The listing builds one solid part. Answer for the finished solid, in the listing's coordinates (mm). Coordinates: 2 decimals unless noted, no trailing zeros. Order: outer loops, then holes, each group sorted by start corner. A loop starts at its lowest first (then second) coordinate and runs counter-clockwise, first axis right, second up. Notation, with made-up numbers: (47.25, 84.25) - (96.25, 84.25) arc R14 cw to (96.25, 104.25) - close; hole circle Ø10 at (64, 74.5). An arc over 180 degrees is marked (long way). Use one line per item in the form item = value. Start each with the question number.
Item 1: Section B-B, the plane x = -21 is taken. Write down the section's boundary in (y, z).
Item 2: Consider line 1 along Y through (x, z) = (-9, -66). Determine where the line is inside the solid, lowest interval first. Write a range as [from, to].
Item 3: Section A-A, the plane z = -18 is taken. Write down the section's boundary in (x, y), and give its area (3 significant figures).
Item 4: Each of these flat-tipped pins is pushed along its axis until it touches: pin 1 Ø1 at (x, y) = (-38, 51) entering from +Z (3 decimals); pin 2 Ø1.6 at (x, y) = (-38, 50.5) entering from -Z (3 decimals); pin 3 Ø3.5 at (y, z) = (51, -17.5) entering from -X; pin 4 Ø4 at (x, y) = (26, 18.5) entering from +Z. Where does it stop, or does it pass through?
Item 5: Section C-C, the plane z = -51 is taken. Write down the section's boundary in (x, y).
from build123d import *

# Parameters (mm, degrees)
SKETCH2_W           = 88.9
SKETCH2_H           = 98.425
BOSS_EXTRUDE1_DEPTH = 69.85
SKETCH3_W           = 6.235827492
SKETCH3_H           = 6.35
BOSS_EXTRUDE2_DEPTH = 3.175


with BuildPart() as part:
    # Sketch2 → Boss-Extrude1 (new body)
    with BuildSketch(Plane.XY):
        Rectangle(SKETCH2_W, SKETCH2_H)
    extrude(amount=-BOSS_EXTRUDE1_DEPTH)

    # Sketch3 → Boss-Extrude2 (add)
    with BuildSketch(Plane(origin=(0, 49.2125, 0), x_dir=(1, 0, 0), z_dir=(0, 1, 0))):
        with Locations((-36.569586254, 19.05)):
            Rectangle(SKETCH3_W, SKETCH3_H)
        with Locations((36.569586254, 19.05)):
            Rectangle(SKETCH3_W, SKETCH3_H)
    extrude(amount=BOSS_EXTRUDE2_DEPTH)


solid = part.part
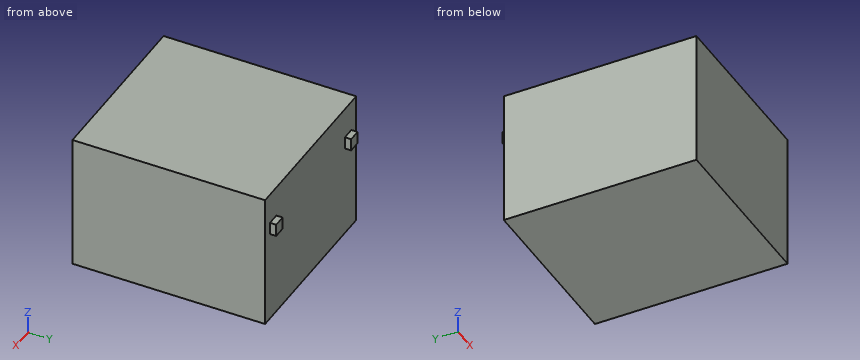
Response:
q1.outline = (-49.21, -69.85) - (49.21, -69.85) - (49.21, 0) - (-49.21, 0) - close
q2.line_1 = [-49.21, 49.21]
q3.outline = (-44.45, -49.21) - (44.45, -49.21) - (44.45, 49.21) - (39.69, 49.21) - (39.69, 52.39) - (33.45, 52.39) - (33.45, 49.21) - (-33.45, 49.21) - (-33.45, 52.39) - (-39.69, 52.39) - (-39.69, 49.21) - (-44.45, 49.21) - close
q3.area = 8,790 mm2
q4.pin_1 = -15.875
q4.pin_2 = -22.225
q4.pin_3 = -39.69
q4.pin_4 = 0
q5.outline = (-44.45, -49.21) - (44.45, -49.21) - (44.45, 49.21) - (-44.45, 49.21) - close
